Could you check a few things on this drawing? It's one solid part, dimensions in mm from its lowest x, y, z. A direction names the side the tool comes from. Round coordinates to 2 decimals unless told otherwise and drop trailing zeros. Write each loop counter-clockwise with the first axis right and the second up, starting at its lowest first coordinate (ties: lowest second). Pieces come first, ordered by that corner, then holes. Notation, with made-up numbers: (17, -28.5) -> (27, -28.5) arc R9 ccw to (27, -22.5) -> close; hole circle Ø4 at (81, 63). An arc over 180 degrees is marked (long way). Return JSON: item names as keys, results as strings.
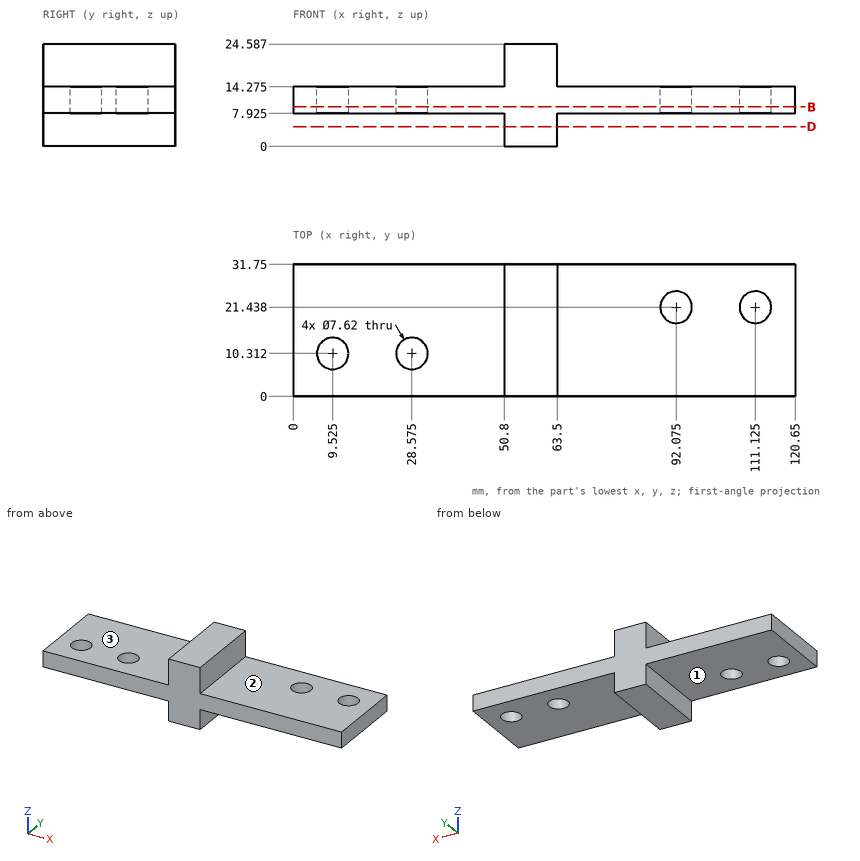
1) Will these pins go through, and if not, where does the flat tip stop? pin 1 Ø10 at (x, y) = (111.12, 21.44) entering from -Z (1 decimal); pin 2 Ø5 at (y, z) = (18, 16) entering from +X; pin 3 Ø8 at (y, z) = (4, 21.5) entering from -X; pin 4 Ø8 at (y, z) = (20.5, 21.5) entering from +X.
Return value:
{"pin 1": "z = 7.9", "pin 2": "x = 120.65", "pin 3": "x = 50.8", "pin 4": "x = 63.5"}
2) If I drill on probe 1 along X at (y, z) = (10.5, 10); probe 2 along X at (y, z) = (2.5, 6); probe 3 along Z at (x, y) = (99, 26.5) (1 decimal), over which ranges is the centre line in solid material (lowest first)? Write a range as [from, to].
Return value:
{"probe 1": "[0, 5.72], [13.33, 24.77], [32.38, 120.65]", "probe 2": "[50.8, 63.5]", "probe 3": "[7.9, 14.3]"}
3) I want a section at D-D, the plane z = 4.75. Please give me the cut outline in (x, y).
Return value:
{"outline": "(50.8, 0) -> (63.5, 0) -> (63.5, 31.75) -> (50.8, 31.75) -> close"}
4) For the marked faces 1, 2 and 3, which set-ups out of +Z, -Z, +X, -X, +Y, -Y let a thin tool reach every point of the face, with its end or its side?
Return value:
{"face 1": "-Z, -X, +Y, -Y", "face 2": "+Z, +X, +Y, -Y", "face 3": "+Z, -X, +Y, -Y"}
5) I want a section at B-B, the plane z = 9.5. Count the separate pieces of the cut face and the enclosed holes in it, and give its area (3 significant figures).
Return value:
{"separate pieces": "1", "enclosed holes": "4", "area": "3,650 mm²"}
